```python
from build123d import *

# Parameters (mm, degrees)
SKETCH1_W           = 95
SKETCH1_H           = 45
BOSS_EXTRUDE1_DEPTH = 25
SKETCH2_R           = 2.5
CUT_EXTRUDE1_DEPTH  = 10
FILLET1_R           = 0.4


with BuildPart() as part:
    # Sketch1 → Boss-Extrude1 (new body)
    with BuildSketch(Plane(origin=(0, 0, 0), x_dir=(1, 0, 0), z_dir=(0, 1, 0))):
        with Locations((47.5, 22.5)):
            Rectangle(SKETCH1_W, SKETCH1_H)
    extrude(amount=BOSS_EXTRUDE1_DEPTH)

    # Sketch2 → Cut-Extrude1 (cut)
    with BuildSketch(Plane(origin=(0, 25, 0), x_dir=(1, 0, 0), z_dir=(0, 1, 0))):
        with Locations(Location((5, 38.75, 0), (0, 0, 270))):
            Circle(SKETCH2_R)
        with Locations(Location((5, 6.25, 0), (0, 0, 270))):
            Circle(SKETCH2_R)
    extrude(amount=-CUT_EXTRUDE1_DEPTH, mode=Mode.SUBTRACT)

    # Fillet1
    fillet1_edges = [part.edges().sort_by_distance(p)[0] for p in [
        (95, 25, -22.5),
        (5, 25, -41.25),
        (47.5, 25, -45),
        (5, 25, -8.75),
        (0, 25, -22.5),
        (47.5, 0, -45),
        (95, 0, -22.5),
        (47.5, 0, 0),
        (0, 0, -22.5),
        (0, 12.5, -45),
        (95, 12.5, -45),
        (95, 12.5, 0),
        (0, 12.5, 0),
        (47.5, 25, 0),
    ]]
    fillet(fillet1_edges, radius=FILLET1_R)


solid = part.part
```
Work out the finished part from the listing and answer in its coordinate system (mm). A direction names the side the tool comes from. Give positions to 0.01 mm unless a question says otherwise; leave off trailing zeros. Write each loop counter-clockwise with the first axis right and the second up, starting at its lowest first coordinate (ties: lowest second). Pieces come first, ordered by that corner, then holes.
(1) Which of the six approach directions +Z, -Z, +X, -X, +Y, -Y give full straight-line access (tool end or side, diameter ignored) to faces 1 (the cylindrical face through (4.04, 19.87, -36.44)), 2 (the flat face through (47, 25, -23))?
Final values:
face 1: +Y
face 2: +Z, -Z, +X, -X, +Y
(2) The part is cut by section B-B on z = -38.75. Write down the section's boundary in (x, y).
Final values:
outline: (0, 0.4) arc R0.4 ccw to (0.4, 0) - (94.6, 0) arc R0.4 ccw to (95, 0.4) - (95, 24.6) arc R0.4 ccw to (94.6, 25) - (7.9, 25) arc R0.4 ccw to (7.5, 24.6) - (7.5, 15) - (2.5, 15) - (2.5, 24.6) arc R0.4 ccw to (2.1, 25) - (0.4, 25) arc R0.4 ccw to (0, 24.6) - close
(3) A straight line is drawn through the part: line 1 (X direction, y = 22, z = -6.25). Find the intervals that lie inside material, in ascending order.
Final values:
line 1: x = 0 to 2.5, 7.5 to 95
(4) The part is cut by section A-A on x = 5. Write down the section's boundary in (y, z), plus the area to 3 significant figures.
Final values:
outline: (0, -44.6) arc R0.4 ccw to (0.4, -45) - (24.6, -45) arc R0.4 ccw to (25, -44.6) - (25, -41.65) arc R0.4 ccw to (24.6, -41.25) - (15, -41.25) - (15, -36.25) - (24.6, -36.25) arc R0.4 ccw to (25, -35.85) - (25, -9.15) arc R0.4 ccw to (24.6, -8.75) - (15, -8.75) - (15, -3.75) - (24.6, -3.75) arc R0.4 ccw to (25, -3.35) - (25, -0.4) arc R0.4 ccw to (24.6, 0) - (0.4, 0) arc R0.4 ccw to (0, -0.4) - close
area: 1,020 mm2
(5) The mould has two halves that part along Z. Classify faces 3 (the flat face through (5, 15, -39)), 4 (the flat face through (47, 12, -45)), 5 (the flat face through (95, 12, -22)): pulls with the +Z half, pulls with the -Z half, needs draft (parallel to the pull), parting line crosses it, or undercut.
Final values:
face 3: undercut
face 4: pulls with the -Z half
face 5: needs draft
(6) A flat-ended cylindrical pin translates along its axis: pin 1 Ø4.5 at (x, z) = (5, -38.75) entering from +Y. Find the tip coordinate at first contact, or state that the pin passes through.
Final values:
pin 1: stops at y = 15
